Source: CAD feature listing. Evaluate the final solid. Frame: model axes, mm. A direction names the side the tool comes from. Round coordinates to 2 decimals unless told otherwise and drop trailing zeros. Write each loop counter-clockwise with the first axis right and the second up, starting at its lowest first coordinate (ties: lowest second). Pieces come first, ordered by that corner, then holes. Notation, with made-up numbers: (-18.5, 53) -> (24.5, 53) arc R23 cw to (24.5, 86) -> close; hole circle Ø11 at (28, -40). An arc over 180 degrees is marked (long way). Put each result on its own line as item: value.
Autodesk Inventor part; units mm, degrees
ref_plane "YZ Plane" through (0, 0, 0) normal (1, 0, 0) x (0, 1, 0)
ref_plane "XZ Plane" through (0, 0, 0) normal (0, 1, 0) x (-1, 0, 0)
ref_plane "XY Plane" through (0, 0, 0) normal (0, 0, 1) x (1, 0, 0)
ref_plane "Arbeitsebene1" through (0, 0, 0) normal (0, 0, 1) x (1, 0, 0)
ref_plane "Arbeitsebene2" through (-1.5, 28.05, 3) normal (0, 0, 1) x (0, -1, 0)
sketch "Skizze2" plane through (-1.5, 28.05, 3) normal (0, 0, 1) x (0, -1, 0)
  circle A0 centre (56.1, 0) radius 4 construction
  circle A1 centre (56.1, 0) radius 3.65
  circle A2 centre (37.4, 0) radius 4 construction
  circle A3 centre (18.7, 0) radius 4 construction
  line L0 (6.2, -3) -> (-6.2, -3) construction
  circle A4 centre (0, 0) radius 4 construction
  circle A5 centre (37.4, 0) radius 3.6
  circle A6 centre (18.7, 0) radius 3.6
  circle A7 centre (0, 0) radius 3.6
  circle A8 centre (66, 1.5) radius 1.4 construction
  circle A9 centre (46.75, 1.5) radius 1.4 construction
  circle A10 centre (28.05, 1.5) radius 1.4 construction
  circle A11 centre (9.35, 1.5) radius 1.4 construction
  circle A12 centre (-9.9, 1.5) radius 1.4 construction
  circle A13 centre (66, 1.5) radius 1.6
  circle A14 centre (46.75, 1.5) radius 1.6
  circle A15 centre (28.05, 1.5) radius 1.6
  circle A16 centre (9.35, 1.5) radius 1.6
  circle A17 centre (-9.9, 1.5) radius 1.6
  line L1 (6, 6) -> (6, -6)
  line L2 (-6, 6) -> (6, 6)
  line L3 (-6, -6) -> (-6, 6)
  line L4 (6, -6) -> (-6, -6)
  circle A18 centre (0, 0) radius 4
  line L5 (62.1, 6) -> (62.1, -6)
  line L6 (50.1, 6) -> (62.1, 6)
  line L7 (50.1, -6) -> (50.1, 6)
  line L8 (62.1, -6) -> (50.1, -6)
  circle A19 centre (56.1, 0) radius 4
  line L9 (69.1, 6) -> (-12.4207, 6)
  line L10 (-12.4207, 6) -> (-12.4207, -6)
  line L11 (-12.4207, -6) -> (69.1, -6)
  line L12 (69.1, -6) -> (69.1, 6)
  point P0 (28.05, 1.5)
  point P1 (50.1, 6)
  point P2 (6, 6)
  point P3 (6, -6)
  dimension "d0" = 7.3
  dimension "d1" = 7.2
  dimension "d2" = 7.2
  dimension "d3" = 7.2
  dimension "d4" = 3.2
  dimension "d5" = 3.2
  dimension "d6" = 3.2
  dimension "d7" = 3.2
  dimension "d8" = 3.2
  dimension "d9" = 7
extrude "Extrusion1" add sketch "Skizze2" along normal blind 10 contours L9 L7 L11 L1 | L1 L4 L3 L2 | L6 L5 L8 L7 | A18 | A19
sketch "Skizze3" plane through (-1.5, 28.05, 13) normal (0, 0, 1) x (1, 0, 0)
  line L0 (-6, 6) -> (-6, -62.1)
  line L1 (-6, -62.1) -> (6, -62.1)
  line L2 (6, -62.1) -> (6, 6)
  line L3 (6, 6) -> (-6, 6)
  circle A0 centre (1.5, -9.35) radius 1.6
  circle A1 centre (1.5, -28.05) radius 1.6
  circle A2 centre (1.5, -46.75) radius 1.6
  circle A3 centre (0, -18.7) radius 3.6
  circle A4 centre (0, -37.4) radius 3.6
  circle A5 centre (0, 0) radius 3.6
  circle A6 centre (0, -56.1) radius 3.35
  circle A7 centre (0, -37.4) radius 3.6
  circle A8 centre (0, -37.4) radius 3.35
  circle A9 centre (0, -18.7) radius 3.6
  circle A10 centre (0, -18.7) radius 3.35
  circle A11 centre (0, 0) radius 3.35
  point P0 (1.5, -28.05)
  dimension "d12" = 6.7
  dimension "d13" = 6.7
  dimension "d14" = 6.7
  dimension "d15" = 6.7
extrude "Extrusion2" add sketch "Skizze3" along normal blind 5 contours L3 L2 L1 L0 | A3 | A4 | A5
sketch "Skizze4" plane through (-1.5, 28.05, 18) normal (0, 0, 1) x (1, 0, 0)
  circle A0 centre (1.5, -46.75) radius 1.6
  circle A1 centre (1.5, -28.05) radius 1.6
  circle A2 centre (1.5, -9.35) radius 1.6
  point P0 (1.5, -28.05)
hole "Bohrung1" at (0, -18.7, 18) at (0, 0, 18) at (0, 18.7, 18) direction (0, 0, -1) diameter 3.2 end through all counterbore diameter 7 counterbore depth 10
fillet "Rundung1" radius 2 4 edges at (4.5, -34.05, 10.5) (-7.5, -34.05, 10.5) (-7.5, 34.05, 10.5) (4.5, 34.05, 10.5)
properties part number "Omniscope_USBC_Bar_lenses"
Q1. Cut plane C-C on y = -28.05. Output: boundary loops of the cut face in (x, z), and give its area (3 significant figures).
Ans:
outline: (-7.5, 3) -> (-5.15, 3) -> (-5.15, 13) -> (-4.85, 13) -> (-4.85, 18) -> (-7.5, 18) -> close; (1.85, 13) -> (2.15, 13) -> (2.15, 3) -> (4.5, 3) -> (4.5, 18) -> (1.85, 18) -> close
area: 73.5 mm^2
Q2. Cut plane D-D on z = 12. Output: boundary loops of the cut face in (x, y).
Ans:
outline: (-7.5, -32.05) arc R2 ccw to (-5.5, -34.05) -> (2.5, -34.05) arc R2 ccw to (4.5, -32.05) -> (4.5, 32.05) arc R2 ccw to (2.5, 34.05) -> (-5.5, 34.05) arc R2 ccw to (-7.5, 32.05) -> close; hole circle Ø7.3 at (-1.5, -28.05); hole circle Ø7.2 at (-1.5, -9.35); hole circle Ø7.2 at (-1.5, 9.35); hole circle Ø7.2 at (-1.5, 28.05); hole circle Ø7 at (0, -18.7); hole circle Ø7 at (0, 0); hole circle Ø7 at (0, 18.7)
Q3. Reachability of faces 4 (the flat face through (-2, 34.05, 10)), 5 (the flat face through (2, -19, 8)), 6 (the cylindrical face through (-2.581, 5.916, 7.93)) from +Z, -Z, +X, -X, +Y, -Y: full face, straight path, thin tool, end or side. Return the list, or none.
Ans:
face 4: +Z, -Z, +X, -X, +Y
face 5: +Z
face 6: -Z
Q4. Draft query along X for faces 1 (the flat face through (-4, 0, 18)), 2 (the cylindrical face through (-6.9, 33.48, 10.6)), 3 (the cylindrical face through (3.105, 17.085, 12.93)). Return one class per face: +X half, -X half, draft (parallel to the pull), parting line (faces both ways), or undercut.
Ans:
face 1: draft
face 2: -X half
face 3: undercut
Q5. Pin query (flat end, axial travel): pin 1 (2 mm diameter, centred on x = 0, y = -1, fed in from +Z). Return the tip coordinate at first contact, or that it passes through.
Ans:
pin 1: stops at z = 8
Q6. Cut plane B-B on z = 15. Output: boundary loops of the cut face in (x, y).
Ans:
outline: (-7.5, -32.05) arc R2 ccw to (-5.5, -34.05) -> (2.5, -34.05) arc R2 ccw to (4.5, -32.05) -> (4.5, 32.05) arc R2 ccw to (2.5, 34.05) -> (-5.5, 34.05) arc R2 ccw to (-7.5, 32.05) -> close; hole circle Ø6.7 at (-1.5, -28.05); hole circle Ø6.7 at (-1.5, -9.35); hole circle Ø6.7 at (-1.5, 9.35); hole circle Ø6.7 at (-1.5, 28.05); hole circle Ø7 at (0, -18.7); hole circle Ø7 at (0, 0); hole circle Ø7 at (0, 18.7)
Q7. Cut plane A-A on y = -18.7. Output: boundary loops of the cut face in (x, z).
Ans:
outline: (-7.5, 3) -> (-1.6, 3) -> (-1.6, 8) -> (-3.5, 8) -> (-3.5, 18) -> (-7.5, 18) -> close; (1.6, 3) -> (4.5, 3) -> (4.5, 18) -> (3.5, 18) -> (3.5, 8) -> (1.6, 8) -> close
Q8. Material intervals for line 1 (X direction, y = -29.5, z = 12.5); line 2 (X direction, y = 18.7, z = 6.65); line 3 (Y direction, x = 2, z = 15.75), sorted ascending. Write a range as [from, to].
Ans:
line 1: x = [-7.5, -4.85], [1.85, 4.5]
line 2: x = [-7.5, -1.6], [1.6, 4.5]
line 3: y = [-34.05, -21.57], [-15.83, -2.87], [2.87, 15.83], [21.57, 34.05]
